The model under review builds one solid part; all positions refer to its coordinate system, in mm. Face numbers are marked on the shaded views. Coordinates: 2 decimals unless noted, no trailing zeros. Loops run counter-clockwise (first coordinate to the right, second up) from the corner with the lowest first, then second, coordinate; pieces in that order, holes last. Notation, with made-up numbers: M 58.5,29 L 99.5,29 A16 cw 99.5,50 Z; hole C 40.25,5 d7. An arc over 180 degrees is marked long. Use CSV: the item, a comma, the result in double quotes. Start each with the question number.
1. Add section A-A, the plane x = 7.5. State how many separate pieces and enclosed holes the cut face has, then the cut area to 3 significant figures.
2. Add section B-B, the plane y = 0. Write out the cut boundary in (x, z), then the cut area to 3 significant figures.
3. For L1, parallel to Z at x = 5, y = -29.15; L2, parallel to X at y = 21.7, z = -22.5; L3, parallel to Z at x = 6, y = -21, list the stretches that pass through material, from the lowest coordinate up.
4. Clearance check with flat-ended pins moving along their axes: P1, Ø2.5, axis at x = 5, z = -22.5, coming from the +Y side; P2, Ø1.3, axis at y = -24.5, z = -23.5, coming from the +X side. State where each tip first meets the part, or that it passes through.
5. Draft analysis for pull direction Y (two halves, no side actions). For the marked faces 1, 2, 3 and 4, state which applies: +Y half, -Y half, draft (parallel to the pull), parting line (faces both ways), or undercut.
6. Add section D-D, the plane z = -4. Write out the cut boundary in (x, y), then the cut area to 3 significant figures.
from build123d import *

# Parameters (mm, degrees)
SKETCH1_W           = 55
SKETCH1_H           = 60
BOSS_EXTRUDE1_DEPTH = 10
SKETCH2_R           = 1.7
CUT_EXTRUDE1_DEPTH  = 10
CUT_EXTRUDE2_START  = -10
SKETCH3_R           = 1.7
CUT_EXTRUDE2_DEPTH  = 10
SKETCH4_W           = 5.8
SKETCH4_H           = 2.6
CUT_EXTRUDE3_DEPTH  = 9
SKETCH5_R           = 8.15
CUT_EXTRUDE4_DEPTH  = 24
SKETCH6_R           = 9.1
CUT_EXTRUDE5_DEPTH  = 1.4
FILLET1_R           = 1
SKETCH7_R           = 1.7
CUT_EXTRUDE6_DEPTH  = 27


with BuildPart() as part:
    # Sketch1 → Boss-Extrude1 (new body)
    with BuildSketch(Plane(origin=(0, 0, 0), x_dir=(0, 0, -1), z_dir=(1, 0, 0))):
        Rectangle(SKETCH1_W, SKETCH1_H)
    extrude(amount=BOSS_EXTRUDE1_DEPTH)

    # Sketch2 → Cut-Extrude1 (cut)
    with BuildSketch(Plane(origin=(0, 30, 0), x_dir=(1, 0, 0), z_dir=(0, 1, 0))):
        with Locations(Location((5, 22.5, 0), (0, 0, 270))):
            Circle(SKETCH2_R)
        with Locations(Location((5, -22.5, 0), (0, 0, 270))):
            Circle(SKETCH2_R)
    extrude(amount=-CUT_EXTRUDE1_DEPTH, mode=Mode.SUBTRACT)

    # Sketch3 → Cut-Extrude2 (cut)
    with BuildSketch(Plane.XZ.offset(30).offset(CUT_EXTRUDE2_START)):
        with Locations(Location((5, 22.5, 0), (0, 0, 90))):
            Circle(SKETCH3_R)
        with Locations(Location((5, -22.5, 0), (0, 0, 90))):
            Circle(SKETCH3_R)
    extrude(amount=CUT_EXTRUDE2_DEPTH, mode=Mode.SUBTRACT)

    # Sketch4 → Cut-Extrude3 (cut)
    with BuildSketch(Plane(origin=(10, 0, 0), x_dir=(0, 0, -1), z_dir=(1, 0, 0))):
        with Locations((-22.5, 25)):
            Rectangle(SKETCH4_W, SKETCH4_H)
        with Locations((22.5, 25)):
            Rectangle(SKETCH4_W, SKETCH4_H)
        with Locations((-22.5, -25)):
            Rectangle(SKETCH4_W, SKETCH4_H)
        with Locations((22.5, -25)):
            Rectangle(SKETCH4_W, SKETCH4_H)
    extrude(amount=-CUT_EXTRUDE3_DEPTH, mode=Mode.SUBTRACT)

    # Sketch5 → Cut-Extrude4 (cut)
    with BuildSketch(Plane(origin=(10, 0, 0), x_dir=(0, 0, -1), z_dir=(1, 0, 0))):
        Circle(SKETCH5_R)
    extrude(amount=-CUT_EXTRUDE4_DEPTH, mode=Mode.SUBTRACT)

    # Sketch6 → Cut-Extrude5 (cut)
    with BuildSketch(Plane(origin=(10, 0, 0), x_dir=(0, 0, -1), z_dir=(1, 0, 0))):
        Circle(SKETCH6_R)
    extrude(amount=-CUT_EXTRUDE5_DEPTH, mode=Mode.SUBTRACT)

    # Fillet1
    fillet1_edges = [part.edges().sort_by_distance(p)[0] for p in [
        (10, 0, 27.5),
        (10, -30, 0),
        (10, 0, -27.5),
        (0, -30, 0),
        (0, 0, 27.5),
        (0, 30, 0),
        (0, 0, -27.5),
        (5, -30, -27.5),
        (5, -30, 27.5),
        (5, 30, 27.5),
        (5, 30, -27.5),
        (10, 30, 0),
    ]]
    fillet(fillet1_edges, radius=FILLET1_R)

    # Sketch7 → Cut-Extrude6 (cut)
    with BuildSketch(Plane(origin=(10, 0, 0), x_dir=(0, 0, -1), z_dir=(1, 0, 0))):
        with Locations((-8.025, 8.03)):
            Circle(SKETCH7_R)
        with Locations((8.025, 8.03)):
            Circle(SKETCH7_R)
        with Locations((8.025, -8.03)):
            Circle(SKETCH7_R)
        with Locations((-8.025, -8.03)):
            Circle(SKETCH7_R)
    extrude(amount=-CUT_EXTRUDE6_DEPTH, mode=Mode.SUBTRACT)


solid = part.part
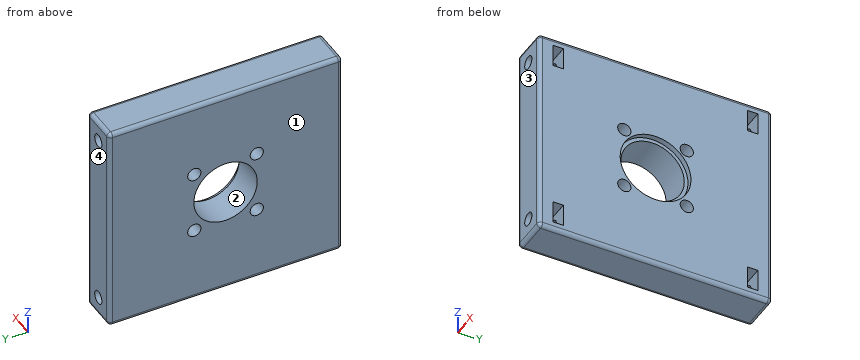
Computed:
1,separate pieces,"1"
1,enclosed holes,"9"
1,area,"2,990 mm^2"
2,outline,"M 0,-26.5 A1 ccw 1,-27.5 L 9,-27.5 A1 ccw 10,-26.5 L 10,-9.1 L 8.6,-9.1 L 8.6,-8.15 L 0,-8.15 Z; M 0,8.15 L 8.6,8.15 L 8.6,9.1 L 10,9.1 L 10,26.5 A1 ccw 9,27.5 L 1,27.5 A1 ccw 0,26.5 Z"
2,area,"383 mm^2"
3,L1,"z = -27.49 to -24.2, -20.8 to 20.8, 24.2 to 27.49"
3,L2,"x = 0 to 3.3, 6.7 to 10"
3,L3,"z = -27.5 to -23.87, -21.13 to 21.13, 23.87 to 27.5"
4,P1,"stops at y = 20"
4,P2,"stops at x = 1"
5,face 1,"draft"
5,face 2,"undercut"
5,face 3,"-Y half"
5,face 4,"+Y half"
6,outline,"M 0,-29 A1 ccw 1,-30 L 9,-30 A1 ccw 10,-29 L 10,-8.17 L 8.6,-8.17 L 8.6,-7.1 L 0,-7.1 Z; M 0,7.1 L 8.6,7.1 L 8.6,8.17 L 10,8.17 L 10,29 A1 ccw 9,30 L 1,30 A1 ccw 0,29 Z"
6,area,"454 mm^2"
